from build123d import *

# Parameters (mm, degrees)
BOSS_EXTRUDE1_DEPTH = 50.5
SKETCH2_R           = 20
BOSS_EXTRUDE2_DEPTH = 26
SKETCH4_W           = 19
SKETCH4_H           = 19
CUT_EXTRUDE1_DEPTH  = 30
SKETCH5_W           = 19
SKETCH5_H           = 19
CUT_EXTRUDE2_DEPTH  = 30


with BuildPart() as part:
    # Sketch1 → Boss-Extrude1 (new body)
    with BuildSketch(Plane(origin=(0, 0, 0), x_dir=(0, 0, -1), z_dir=(1, 0, 0))):
        Polygon((-12, 0), (12, 0), (22.5, 23.8), (50, 23.8), (50, 7.8), (35, -26.2), (-35, -26.2), (-50, 7.8), (-50, 23.8), (-22.5, 23.8), align=None)
    extrude(amount=-BOSS_EXTRUDE1_DEPTH)

    # Sketch2 → Boss-Extrude2 (add)
    with BuildSketch(Plane.XZ.offset(26.2)):
        with Locations(Location((-25.25, 0, 0), (0, 0, 90))):
            Circle(SKETCH2_R)
    extrude(amount=BOSS_EXTRUDE2_DEPTH)

    # Sketch4 → Cut-Extrude1 (cut)
    with BuildSketch(Plane.XY.offset(50)):
        with Locations((-25.25, -16.7)):
            Rectangle(SKETCH4_W, SKETCH4_H)
    extrude(amount=-CUT_EXTRUDE1_DEPTH, mode=Mode.SUBTRACT)

    # Sketch5 → Cut-Extrude2 (cut)
    with BuildSketch(Plane(origin=(0, 0, -50), x_dir=(-1, 0, 0), z_dir=(0, 0, -1))):
        with Locations((25.25, -16.7)):
            Rectangle(SKETCH5_W, SKETCH5_H)
    extrude(amount=-CUT_EXTRUDE2_DEPTH, mode=Mode.SUBTRACT)


solid = part.part
The model under review builds one solid part; all positions refer to its coordinate system, in mm. A direction names the side the tool comes from. Give positions to 0.01 mm unless a question says otherwise; leave off trailing zeros. Order: outer loops, then holes, each group sorted by start corner. A loop starts at its lowest first (then second) coordinate and runs counter-clockwise, first axis right, second up. Notation, with made-up numbers: M -36,41.25 L -1,41.25 A22 ccw -1,70.25 Z; hole C -32.5,-30.75 d2. An arc over 180 degrees is marked long. Use one line per item in the form item = value. Start each with the question number.
Item 1: We need section B-B on z = 0. Give the boundary of the cut face in (x, y), plus the area to 3 significant figures.
Item 2: We need section D-D on y = -35.5. Give the boundary of the cut face in (x, z), plus the area to 3 significant figures.
Item 3: We need section C-C on x = -31. Give the boundary of the cut face in (y, z), plus the area to 3 significant figures.
Item 4: We need section A-A on y = 18. Give the boundary of the cut face in (x, z).
Item 5: For faces 1 (the flat face through (-25, -7.2, -32)), 2 (the flat face through (-4, -26.2, 0)), 3 (the flat face through (-24.896, 12.067, 17.324)), 4 (the flat face through (-25, 23.8, -36)), 5 (the flat face through (-34.75, -17, 29)), list the 3-axis set-ups (+Z, -Z, +X, -X, +Y, -Y) from which the entire face can be reached by the end or side of a thin tool; tool diameter is ignored.
Item 6: Insertion check: pin 1 Ø5.5 at (x, y) = (-27.5, -16) entering from -Z; pin 2 Ø5.5 at (x, y) = (-21.5, -20.5) entering from +Z; pin 3 Ø10 at (x, z) = (-28.5, -0.5) entering from +Y; pin 4 Ø9.5 at (y, z) = (-16.5, -36.5) entering from +X. Each pin has a flat end and moves straight along its axis. Give the tip position at first contact, or say it passes through.
Item 7: To check wall thickness, follow line 1 along X through (y, z) = (-10, 27); line 2 along Y through (x, z) = (-34.5, -38); line 3 along Y through (x, z) = (-41.5, 27). State the ranges of each line that lie inside material, in increasing order. Write a range as from..to.
Item 8: The part is to be moulded in two halves that separate along Z. For faces 6 (the flat face through (-25, 0, 0)), 7 (the cylindrical face through (-5.726, -39.018, -4.336)), 8 (the flat face through (-15.75, -17, 29)), say which applies: pulls with the +Z half, pulls with the -Z half, needs draft (parallel to the pull), parting line crosses it, or undercut.
Completed:
q1.outline = M -50.5,-26.2 L -45.25,-26.2 L -45.25,-52.2 L -5.25,-52.2 L -5.25,-26.2 L 0,-26.2 L 0,0 L -50.5,0 Z
q1.area = 2,360 mm²
q2.outline = C -25.25,0 d40
q2.area = 1,260 mm²
q3.outline = M -52.2,-19.16 L -26.2,-19.16 L -26.2,-20 L -7.2,-20 L -7.2,-43.38 L 7.8,-50 L 23.8,-50 L 23.8,-22.5 L 0,-12 L 0,12 L 23.8,22.5 L 23.8,50 L 7.8,50 L -7.2,43.38 L -7.2,20 L -26.2,20 L -26.2,19.16 L -52.2,19.16 Z
q3.area = 3,940 mm²
q4.outline = M -50.5,-50 L 0,-50 L 0,-19.94 L -50.5,-19.94 Z; M -50.5,19.94 L 0,19.94 L 0,50 L -50.5,50 Z
q5.face_1 = -Z, -Y
q5.face_2 = +X, -Y
q5.face_3 = +X, -X, +Y
q5.face_4 = +Z, -Z, +X, -X, +Y
q5.face_5 = +Z, -Y
q6.pin_1 = -20
q6.pin_2 = 20
q6.pin_3 = 0
q6.pin_4 = 0
q7.line_1 = -50.5..-34.75, -15.75..0
q7.line_2 = -7.2..23.8
q7.line_3 = -26.2..23.8
q8.face_6 = undercut
q8.face_7 = parting line crosses it
q8.face_8 = needs draft
